Verification items for the finished model (mm, model axes). A direction names the side the tool comes from. Coordinates: 2 decimals unless noted, no trailing zeros. Write each loop counter-clockwise with the first axis right and the second up, starting at its lowest first coordinate (ties: lowest second). Pieces come first, ordered by that corner, then holes. Notation, with made-up numbers: (20.25, 62) -> (60.25, 62) arc R30 cw to (60.25, 101) -> close; hole circle Ø11 at (-27, 73.25). An arc over 180 degrees is marked (long way). Answer in a Markdown table with one row per item.
```python
from build123d import *

# Parameters (mm, degrees)
CROQUIS1_W                   = 39
CROQUIS1_H                   = 43
CROQUIS1_R                   = 7
CROQUIS1_R_2                 = 1.7
SALIENTE_EXTRUIR1_DEPTH      = 3.6
CROQUIS2_R                   = 2.95
CORTAR_EXTRUIR1_DEPTH        = 1.6
CROQUIS3_W                   = 10
CROQUIS3_H                   = 8.4
SALIENTE_EXTRUIR2_DEPTH      = 8
CROQUIS4_R                   = 1.7
CORTAR_EXTRUIR2_DEPTH        = 11
CORTAR_EXTRUIR3_DEPTH        = 1.5
CORTAR_EXTRUIR3_DEPTH_BACK   = 1.5
SALIENTE_EXTRUIR3_DEPTH      = 12.5
SALIENTE_EXTRUIR3_DEPTH_BACK = 12.5
CORTAR_EXTRUIR4_DEPTH        = 3


with BuildPart() as part:
    # Croquis1 → Saliente-Extruir1 (new body)
    with BuildSketch(Plane(origin=(0, 0, 0), x_dir=(1, 0, 0), z_dir=(0, 1, 0))):
        with Locations((2, -2.205128205)):
            Rectangle(CROQUIS1_W, CROQUIS1_H)
        Circle(CROQUIS1_R, mode=Mode.SUBTRACT)
        with Locations((-15.5, 15.5)):
            Circle(CROQUIS1_R_2, mode=Mode.SUBTRACT)
        with Locations((15.5, 15.5)):
            Circle(CROQUIS1_R_2, mode=Mode.SUBTRACT)
        with Locations((-15.5, -15.5)):
            Circle(CROQUIS1_R_2, mode=Mode.SUBTRACT)
        with Locations((15.5, -15.5)):
            Circle(CROQUIS1_R_2, mode=Mode.SUBTRACT)
    extrude(amount=SALIENTE_EXTRUIR1_DEPTH)

    # Croquis2 → Cortar-Extruir1 (cut)
    with BuildSketch(Plane(origin=(0, 3.6, 0), x_dir=(1, 0, 0), z_dir=(0, 1, 0))):
        with Locations((-15.5, 15.5)):
            Circle(CROQUIS2_R)
        with Locations((15.5, 15.5)):
            Circle(CROQUIS2_R)
        with Locations((-15.5, -15.5)):
            Circle(CROQUIS2_R)
        with Locations((15.5, -15.5)):
            Circle(CROQUIS2_R)
    extrude(amount=-CORTAR_EXTRUIR1_DEPTH, mode=Mode.SUBTRACT)

    # Croquis3 → Saliente-Extruir2 (add)
    with BuildSketch(Plane(origin=(0, 3.6, 0), x_dir=(1, 0, 0), z_dir=(0, 1, 0))):
        with Locations((16.5, -7.3)):
            Rectangle(CROQUIS3_W, CROQUIS3_H)
    extrude(amount=SALIENTE_EXTRUIR2_DEPTH)

    # Croquis4 → Cortar-Extruir2 (cut)
    with BuildSketch(Plane.XY.offset(11.5)):
        with Locations((16.5, 7.6)):
            Circle(CROQUIS4_R)
    extrude(amount=-CORTAR_EXTRUIR2_DEPTH, mode=Mode.SUBTRACT)

    # Croquis5 → Cortar-Extruir3 (cut, two sides)
    with BuildSketch(Plane.XY.offset(7.3)) as cortar_extruir3_sk:
        Polygon((13.598814897, 9.275), (13.598814897, 15.925), (19.401185103, 15.925), (19.401185103, 9.275), (19.401185103, 5.925), (16.5, 4.25), (13.598814897, 5.925), align=None)
    extrude(amount=CORTAR_EXTRUIR3_DEPTH, mode=Mode.SUBTRACT)
    extrude(cortar_extruir3_sk.sketch, amount=-CORTAR_EXTRUIR3_DEPTH_BACK, mode=Mode.SUBTRACT)

    # Croquis6 → Saliente-Extruir3 (add, two sides)
    with BuildSketch(Plane.XY) as saliente_extruir3_sk:
        Polygon((-10.5, 2.456284193), (-14.9, 7.7), (-6.1, 7.7), align=None)
    extrude(amount=SALIENTE_EXTRUIR3_DEPTH)
    extrude(saliente_extruir3_sk.sketch, amount=-SALIENTE_EXTRUIR3_DEPTH_BACK)

    # Croquis7 → Cortar-Extruir4 (cut)
    with BuildSketch(Plane(origin=(0, 3.6, 0), x_dir=(1, 0, 0), z_dir=(0, 1, 0))):
        with BuildLine():
            Line((-17.5, -13.331475156), (-17.5, -17.668524844))
            ThreePointArc((-17.5, -17.668524844), (-12.55, -15.5), (-17.5, -13.331475156))
        make_face()
        with BuildLine():
            Line((-17.5, 17.668524844), (-17.5, 13.331475156))
            ThreePointArc((-17.5, 13.331475156), (-12.55, 15.5), (-17.5, 17.668524844))
        make_face()
    extrude(amount=-CORTAR_EXTRUIR4_DEPTH, mode=Mode.SUBTRACT)


solid = part.part
```
1. Sectioned sample at C-C, the plane z = 15.5. Record the cut outline in (x, y), and give its area (3 significant figures).
Findings below:
| item | result |
|---|---|
| outline | (-17.5, 0) -> (-17.2, 0) -> (-17.2, 0.6) -> (-17.5, 0.6) -> close; (-13.8, 0) -> (13.8, 0) -> (13.8, 2) -> (12.55, 2) -> (12.55, 3.6) -> (-12.55, 3.6) -> (-12.55, 0.6) -> (-13.8, 0.6) -> close; (17.2, 0) -> (21.5, 0) -> (21.5, 3.6) -> (18.45, 3.6) -> (18.45, 2) -> (17.2, 2) -> close |
| area | 107 mm² |
2. Sectioned sample at A-A, the plane x = 0. Record the cut outline in (y, z).
Findings below:
| item | result |
|---|---|
| outline | (0, -19.29) -> (3.6, -19.29) -> (3.6, -7) -> (0, -7) -> close; (0, 7) -> (3.6, 7) -> (3.6, 23.71) -> (0, 23.71) -> close |
3. Material ranges on probe 1 along X at (y, z) = (0.2, -15.5); probe 2 along Z at (x, y) = (-15.5, 2.7); probe 3 along Z at (x, y) = (15.5, 1.15), recorded low to high. Write a range as from..to.
Findings below:
| item | result |
|---|---|
| probe 1 | x = -17.5..-17.2, -13.8..13.8, 17.2..21.5 |
| probe 2 | z = -19.29..-18.45, -12.55..12.55, 18.45..23.71 |
| probe 3 | z = -19.29..-17.2, -13.8..13.8, 17.2..23.71 |
4. Sectioned sample at D-D, the plane x = -15.5. Record the cut outline in (y, z), and give its area (3 significant figures).
Findings below:
| item | result |
|---|---|
| outline | (0, -19.29) -> (3.6, -19.29) -> (3.6, -18.45) -> (0.6, -18.45) -> (0.6, -17.2) -> (0, -17.2) -> close; (0, -13.8) -> (0.6, -13.8) -> (0.6, -12.55) -> (3.6, -12.55) -> (3.6, 12.55) -> (0.6, 12.55) -> (0.6, 13.8) -> (0, 13.8) -> close; (0, 17.2) -> (0.6, 17.2) -> (0.6, 18.45) -> (3.6, 18.45) -> (3.6, 23.71) -> (0, 23.71) -> close |
| area | 115 mm² |
5. Sectioned sample at B-B, the plane z = 0. Record the cut outline in (x, y), and give its area (3 significant figures).
Findings below:
| item | result |
|---|---|
| outline | (-17.5, 0) -> (-7, 0) -> (-7, 3.6) -> (-9.54, 3.6) -> (-6.1, 7.7) -> (-14.9, 7.7) -> (-11.46, 3.6) -> (-17.5, 3.6) -> close; (7, 0) -> (21.5, 0) -> (21.5, 3.6) -> (7, 3.6) -> close |
| area | 112 mm² |
6. Go/stop test with flat-tipped pins: pin 1 (6.5 mm diameter, centred on x = 14.5, z = -16, fed in from +Y); pin 2 (16 mm diameter, centred on x = 0, z = 0, fed in from +Y); pin 3 (6.5 mm diameter, centred on x = 15.5, y = 9.5, fed in from -Z). Record where each tip stops, or that it passes through.
Findings below:
| item | result |
|---|---|
| pin 1 | stops at y = 3.6 |
| pin 2 | stops at y = 7.7 |
| pin 3 | stops at z = 3.1 |
7. Release check for a two-part mould opening along X. For faces 1 (the face through (16, 11.6, 5)), 2 (the face through (-7.796, 5.679, 0.175)), 3 (the face through (-17.5, 2, 3)) record: released by +X, released by -X, zero draft, split by the parting line, or undercut.
Findings below:
| item | result |
|---|---|
| face 1 | zero draft |
| face 2 | undercut |
| face 3 | released by -X |
8. Access from +Z, -Z, +X, -X, +Y, -Y to the whole of each face (thin tool, end or side, straight path). Record for faces 4 (the face through (-10, 6, -12.5)), 5 (the face through (12.553, 2.811, 15.37)), 6 (the face through (2, 2, 23.705)), 7 (the face through (-11, 7.7, 0)).
Findings below:
| item | result |
|---|---|
| face 4 | -Z, +X, -X, +Y |
| face 5 | +Y |
| face 6 | +Z, +X, -X, +Y, -Y |
| face 7 | +Z, -Z, -X, +Y |
